```python
from build123d import *

# Parameters (mm, degrees)
SKETCH1_W           = 76.2
SKETCH1_H           = 2.54
BOSS_EXTRUDE1_DEPTH = 7.62
SKETCH3_W           = 2.54
SKETCH3_H           = 2.54
BOSS_EXTRUDE2_DEPTH = 7.62
SKETCH4_W           = 15.24
SKETCH4_H           = 2.54
BOSS_EXTRUDE3_DEPTH = 5.08
SKETCH5_W           = 1.27
SKETCH5_H           = 2.54
CUT_EXTRUDE2_DEPTH  = 8.89


with BuildPart() as part:
    # Sketch1 → Boss-Extrude1 (new body)
    with BuildSketch(Plane.XY):
        with Locations((38.1, 1.27)):
            Rectangle(SKETCH1_W, SKETCH1_H)
    extrude(amount=BOSS_EXTRUDE1_DEPTH)

    # Sketch3 → Boss-Extrude2 (add)
    with BuildSketch(Plane.ZY):
        with Locations((1.27, 1.27)):
            Rectangle(SKETCH3_W, SKETCH3_H)
    extrude(amount=BOSS_EXTRUDE2_DEPTH)

    # Sketch4 → Boss-Extrude3 (add)
    with BuildSketch(Plane(origin=(0, 0, 0), x_dir=(-1, 0, 0), z_dir=(0, 0, -1))):
        with Locations((-77.47, 1.27)):
            Rectangle(SKETCH4_W, SKETCH4_H)
    extrude(amount=BOSS_EXTRUDE3_DEPTH)

    # Sketch5 → Cut-Extrude2 (cut)
    with BuildSketch(Plane(origin=(85.09, 0, 0), x_dir=(0, 0, -1), z_dir=(1, 0, 0))):
        with Locations((0.635, 1.27)):
            Rectangle(SKETCH5_W, SKETCH5_H)
    extrude(amount=-CUT_EXTRUDE2_DEPTH, mode=Mode.SUBTRACT)


solid = part.part
```
The listing builds one solid part. Answer for the finished solid, in the listing's coordinates (mm). A direction names the side the tool comes from. Give positions to 0.01 mm unless a question says otherwise; leave off trailing zeros. Loops run counter-clockwise (first coordinate to the right, second up) from the corner with the lowest first, then second, coordinate; pieces in that order, holes last. Notation, with made-up numbers: (43.25, 33.5) - (89.25, 33.5) arc R26 ccw to (89.25, 57.5) - close; hole circle Ø8 at (-12, 26). An arc over 180 degrees is marked (long way). Return JSON: item names as keys, results as strings. Group by question number.
1. Find section A-A (y = 2). Write down the section's boundary in (x, z).
2. Find section C-C (x = 24.5). Write down the section's boundary in (y, z).
3. Straight lines are drawn through the part: line 1 (Z direction, x = 37, y = 2.3); line 2 (X direction, y = 2.2, z = -4.5); line 3 (Z direction, x = -1, y = 0.55). For each, find the intervals that lie inside material, in ascending order. Write a range as [from, to].
4. Given pin 1 Ø1.5 at (y, z) = (2, 5.5) entering from +X; pin 2 Ø1.3 at (y, z) = (1, 5.5) entering from -X; pin 3 Ø1.3 at (x, y) = (28.5, 1) entering from -Z, each flat-ended and moving along its own axis, determine where each tip first touches the part or whether it passes through.
5. Find section B-B (z = 1). Write down the section's boundary in (x, y), then the cut area to 3 significant figures.
6. Which of the six approach directions +Z, -Z, +X, -X, +Y, -Y give full straight-line access (tool end or side, diameter ignored) to faces 1 (the flat face through (-4, 1, 2.54)), 2 (the flat face through (69.85, 1, -3)), 3 (the flat face through (76.2, 1, 3))?
Verdict:
{
 "1": {"outline": "(-7.62, 0) - (69.85, 0) - (69.85, -5.08) - (85.09, -5.08) - (85.09, -1.27) - (76.2, -1.27) - (76.2, 7.62) - (0, 7.62) - (0, 2.54) - (-7.62, 2.54) - close"},
 "2": {"outline": "(0, 0) - (2.54, 0) - (2.54, 7.62) - (0, 7.62) - close"},
 "3": {"line 1": "z = [0, 7.62]", "line 2": "x = [69.85, 85.09]", "line 3": "z = [0, 2.54]"},
 "4": {"pin 1": "stops at x = 76.2", "pin 2": "stops at x = 0", "pin 3": "stops at z = 0"},
 "5": {"outline": "(-7.62, 0) - (76.2, 0) - (76.2, 2.54) - (-7.62, 2.54) - close", "area": "213 mm^2"},
 "6": {"face 1": "+Z, -X, +Y, -Y", "face 2": "-Z, -X, +Y, -Y", "face 3": "+Z, +X, +Y, -Y"}
}
